Part model, mm, in its own coordinate system. Face numbers are marked on the shaded views. A direction names the side the tool comes from. Give positions to 0.01 mm unless a question says otherwise; leave off trailing zeros. Order: outer loops, then holes, each group sorted by start corner. A loop starts at its lowest first (then second) coordinate and runs counter-clockwise, first axis right, second up. Notation, with made-up numbers: M 34,-13.75 L 80,-13.75 A25 ccw 80,16.25 Z; hole C 56,56 d6. An arc over 180 degrees is marked long. Answer as a JSON object with one key per item and string values.
Autodesk Inventor part; units mm, degrees
ref_plane "YZ Plane" through (0, 0, 0) normal (1, 0, 0) x (0, 1, 0)
ref_plane "XZ Plane" through (0, 0, 0) normal (0, 1, 0) x (-1, 0, 0)
ref_plane "XY Plane" through (0, 0, 0) normal (0, 0, 1) x (1, 0, 0)
sketch "Sketch1" plane through (0, 0, 0) normal (0, 0, 1) x (1, 0, 0)
  line L0 (40, 160) -> (876.7461, 160)
  line L1 (876.7461, 160) -> (876.7461, -160)
  line L2 (876.7461, -160) -> (40, -160)
  line L3 (40, -200) -> (40, -160)
  line L4 (916.7461, -200) -> (40, -200)
  line L5 (916.7461, -160) -> (916.7461, -200)
  line L6 (916.7461, 160) -> (916.7461, -160)
  line L7 (916.7461, 200) -> (916.7461, 160)
  line L8 (40, 200) -> (916.7461, 200)
  line L9 (40, 160) -> (40, 200)
  line L10 (618.4585, 200) -> (418.4585, 200)
  line L11 (418.4585, 200) -> (418.4585, 160)
  line L12 (418.4585, 160) -> (618.4585, 160)
  line L13 (618.4585, 160) -> (618.4585, 200)
  line L14 (618.4585, -160) -> (418.4585, -160)
  line L15 (418.4585, -160) -> (418.4585, -200)
  line L16 (418.4585, -200) -> (618.4585, -200)
  line L17 (618.4585, -200) -> (618.4585, -160)
  point P0 (0, 0)
  dimension "d0" = 200
extrude "Extrusion1" add sketch "Sketch1" along normal blind 50 contours L11 L8 L13 L0 | L17 L4 L15 L2
sketch "Sketch2" plane through (418.4585, -160, 0) normal (0, 1, 0) x (1, 0, 0)
  arc A0 (78.7868, -178.7868) -> (121.2132, -178.7868) centre (100, -157.5736) ccw
  arc A1 (78.7868, -178.7868) -> (121.2132, -178.7868) centre (100, -157.5736) ccw
  circle A2 centre (100, -157.5736) radius 10
  line L0 (0, 0) -> (0, -50)
  line L1 (0, 0) -> (200, 0)
  line L2 (200, 0) -> (200, -50)
  line L3 (200, 0) -> (200, -87.5736)
  line L4 (200, 0) -> (170, 0)
  line L5 (170, 0) -> (170, -30)
  line L6 (170, -30) -> (200, -30)
  line L7 (200, -30) -> (200, 0)
  line L8 (0, -50) -> (200, -50)
  point P0 (-418.4585, 0)
  dimension "d7" = 20
  dimension "d10" = 30
  dimension "d11" = 30
extrude "Extrusion2" add sketch "Sketch2" along normal up to next contours L1 L2 L6 L5
sketch "Sketch3" plane through (618.4585, -200, 0) normal (1, 0, 0) x (0, 0, -1)
  line L0 (-30, 40) -> (-30, 360)
  line L1 (-30, 40) -> (-50, 40)
  line L2 (-50, 0) -> (-50, 40)
  line L3 (0, 0) -> (-50, 0)
  line L4 (0, 0) -> (0, 400)
  line L5 (0, 400) -> (-50, 400)
  line L6 (-50, 360) -> (-50, 400)
  line L7 (-30, 360) -> (-50, 360)
  line L8 (-30, 40) -> (-30, 360)
  line L9 (-30, 305) -> (-150, 305)
  arc A0 (-150, 305) -> (-150, 95) centre (-150, 200) ccw
  line L10 (-150, 95) -> (-30, 95)
  line L11 (-30, 305) -> (-30, 95)
  circle A1 centre (-150, 200) radius 85
  point P0 (0, 200)
  point P1 (0, 200)
  dimension "d13" = 170
  dimension "d14" = 20
  dimension "d15" = 120
extrude "Extrusion3" add sketch "Sketch3" against normal blind 30 contours L10 A0 L9 L0
properties part number "emmerhouder"
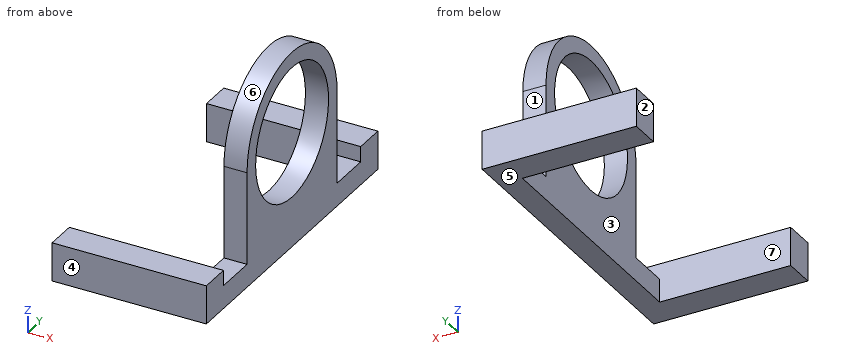
1. Cut at C-C on x = 595. Give the cut face in (y, z), plus the area to 3 significant figures.
Worked answers:
{"outline": "M -200,0 L 200,0 L 200,50 L 160,50 L 160,30 L 105,30 L 105,150 A105 ccw -105,150 L -105,30 L -160,30 L -160,50 L -200,50 Z; hole C 0,150 d170", "area": "33,400 mm^2"}
2. Cut at A-A on x = 535.5. Give the cut face in (y, z), plus the area to 3 significant figures.
Worked answers:
{"outline": "M -200,0 L -160,0 L -160,50 L -200,50 Z; M 160,0 L 200,0 L 200,50 L 160,50 Z", "area": "4,000 mm^2"}
3. Which spindle directions (+Z, -Z, +X, -X, +Y, -Y) get a long thin tool onto all of the face, cutting with end or side? Do the marked faces 1, 2 and 3. Say none if no direction does.
Worked answers:
{"face 1": "+Z, +X, -X", "face 2": "+Z, -Z, -X, +Y, -Y", "face 3": "+Z, -Z, -X"}
4. Probe line 1 along Y through (x, z) = (607, 40.5); line 2 along Y through (x, z) = (611.5, 150); line 3 along Y through (x, z) = (464, 18). List the from-to ranges inside material, lowest first.
Worked answers:
{"line 1": "y = -200 to -160, -105 to 105, 160 to 200", "line 2": "y = -105 to -85, 85 to 105", "line 3": "y = -200 to -160, 160 to 200"}
5. Pin check, flat tips, straight feed: P1, Ø15, axis at x = 607.5, z = 84, coming from the +Y side; P2, Ø10, axis at y = 87.5, z = 208, coming from the -X side; P3, Ø9, axis at x = 606, y = -123.5, coming from the +Z side. Stop position of each tip, or through.
Worked answers:
{"P1": "stops at y = 105", "P2": "stops at x = 588.46", "P3": "stops at z = 30"}
6. Cut at D-D on y = 128. Give the cut face in (x, z), plus the area to 3 significant figures.
Worked answers:
{"outline": "M 588.46,0 L 618.46,0 L 618.46,30 L 588.46,30 Z", "area": "900 mm^2"}
7. Cut at B-B on y = 0. Give the cut face in (x, z).
Worked answers:
{"outline": "M 588.46,0 L 618.46,0 L 618.46,65 L 588.46,65 Z; M 588.46,235 L 618.46,235 L 618.46,255 L 588.46,255 Z"}
8. Two-plate mould, pull along Y, no slides. Class the marked faces 4, 5, 6 and 7: +Y half, -Y half, draft (parallel to the pull), parting line (faces both ways), or undercut.
Worked answers:
{"face 4": "-Y half", "face 5": "draft", "face 6": "parting line", "face 7": "undercut"}
